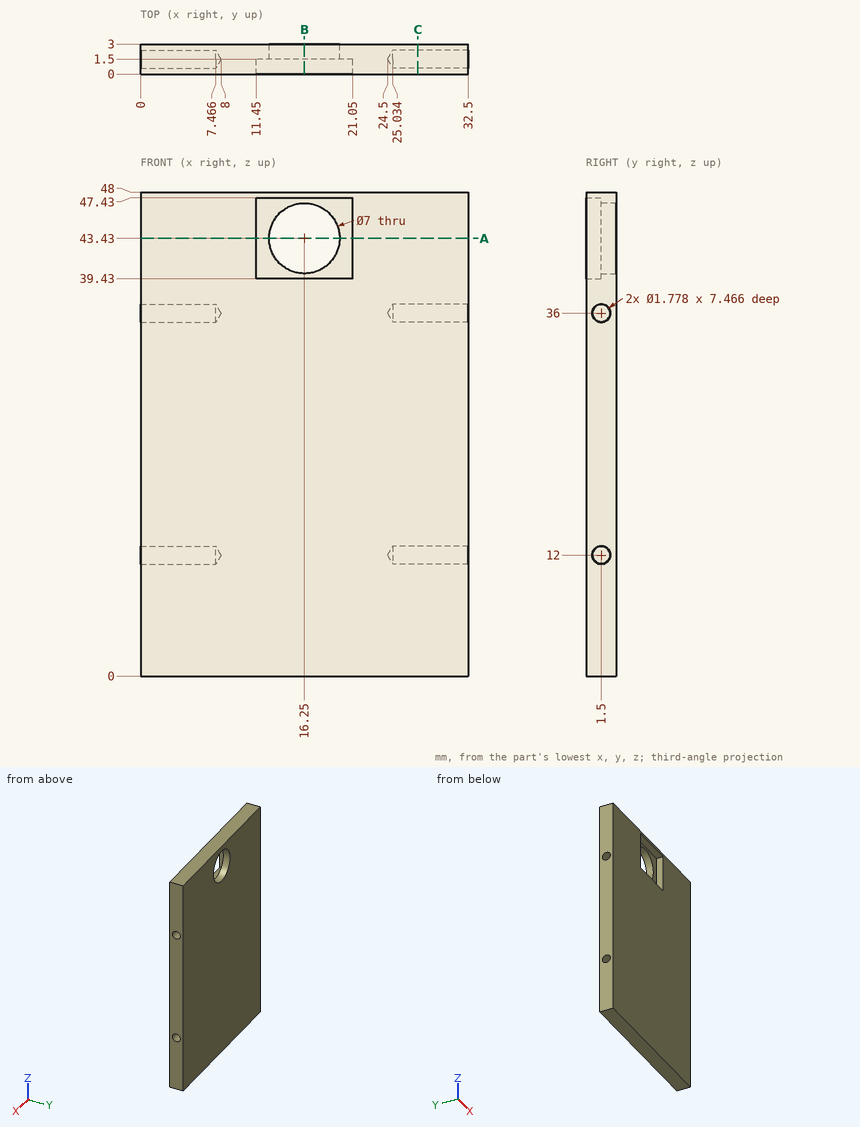
Verification items for this drawing (mm, ordinates from the low corner). Coordinates: 2 decimals unless noted, no trailing zeros. Order: outer loops, then holes, each group sorted by start corner. A loop starts at its lowest first (then second) coordinate and runs counter-clockwise, first axis right, second up.
Q1. Sectioned sample at C-C on x = 27.5. Record the cut outline in (y, z).
Reply:
outline: (0, 0) - (3, 0) - (3, 48) - (0, 48) - close; hole circle Ø1.78 at (1.5, 12); hole circle Ø1.78 at (1.5, 36)
Q2. Sectioned sample at B-B on x = 16.25. Record the cut outline in (y, z).
Reply:
outline: (0, 0) - (3, 0) - (3, 39.93) - (1.5, 39.93) - (1.5, 39.43) - (0, 39.43) - close; (0, 47.43) - (1.5, 47.43) - (1.5, 46.93) - (3, 46.93) - (3, 48) - (0, 48) - close
Q3. Depth check by flat-ended pin: pin 1 Ø1.1 at (y, z) = (1.5, 36) entering from +X. Enter the tip coordinate at first touch or a pass-through.
Reply:
pin 1: stops at x = 24.83
Q4. Thickness scan on probe 1 along Z at (x, y) = (27.75, 1.5); probe 2 along Y at (x, z) = (4.25, 36); probe 3 along Z at (x, y) = (20, 1.3). Record the ranges inside material, lowest first.
Reply:
probe 1: z = 0 to 11.11, 12.89 to 35.11, 36.89 to 48
probe 2: y = 0 to 0.61, 2.39 to 3
probe 3: z = 0 to 39.43, 47.43 to 48
Q5. Sectioned sample at A-A on z = 43.43. Record the cut outline in (x, y).
Reply:
outline: (0, 0) - (11.45, 0) - (11.45, 1.5) - (12.75, 1.5) - (12.75, 3) - (0, 3) - close; (19.75, 1.5) - (21.05, 1.5) - (21.05, 0) - (32.5, 0) - (32.5, 3) - (19.75, 3) - close
